from build123d import *

# Parameters (mm, degrees)
SKETCH1_W           = 21.9
SKETCH1_H           = 28.1
BOSS_EXTRUDE1_DEPTH = 1.75
SKETCH2_R           = 1.4
CUT_EXTRUDE1_DEPTH  = 18.89881281
SKETCH3_W           = 5.2
SKETCH3_H           = 5.2
BOSS_EXTRUDE2_DEPTH = 1
SKETCH4_W           = 20.3
SKETCH4_H           = 2.5
BOSS_EXTRUDE3_DEPTH = 2.55
SKETCH5_W           = 0.6
SKETCH5_H           = 0.6
BOSS_EXTRUDE4_DEPTH = 6.1
LPATTERN1_COUNT     = 8
LPATTERN1_PITCH     = 2.54


with BuildPart() as part:
    # Sketch1 → Boss-Extrude1 (new body)
    with BuildSketch(Plane.XY):
        Rectangle(SKETCH1_W, SKETCH1_H)
    extrude(amount=BOSS_EXTRUDE1_DEPTH)

    # Sketch2 → Cut-Extrude1 (cut, through all)
    with BuildSketch(Plane.XY.offset(1.75)):
        with Locations((-9.075, -0.89)):
            Circle(SKETCH2_R)
        with Locations((9.075, -0.89)):
            Circle(SKETCH2_R)
        with Locations((9.075, -12.05)):
            Circle(SKETCH2_R)
        with Locations((-9.075, -12.05)):
            Circle(SKETCH2_R)
    extrude(amount=-CUT_EXTRUDE1_DEPTH, mode=Mode.SUBTRACT)

    # Sketch3 → Boss-Extrude2 (add)
    with BuildSketch(Plane.XY.offset(1.75)):
        with Locations((0, -6.47)):
            Rectangle(SKETCH3_W, SKETCH3_H)
    extrude(amount=BOSS_EXTRUDE2_DEPTH)

    # Sketch4 → Boss-Extrude3 (add)
    with BuildSketch(Plane.XY.offset(1.75)):
        with Locations((0, 12.3)):
            Rectangle(SKETCH4_W, SKETCH4_H)
    extrude(amount=BOSS_EXTRUDE3_DEPTH)

    # Sketch5 → Boss-Extrude4 (add)
    with BuildSketch(Plane.XY.offset(4.3)):
        with Locations((-8.78, 12.3)):
            Rectangle(SKETCH5_W, SKETCH5_H)
    boss_extrude4 = extrude(amount=BOSS_EXTRUDE4_DEPTH)

    # LPattern1: Boss-Extrude4 ×8
    with Locations(*[(i * LPATTERN1_PITCH, 0, 0) for i in range(1, LPATTERN1_COUNT)]):
        add(boss_extrude4)


solid = part.part
Read the model definition and answer for the solid it produces. Units are mm, in the model's axes. A direction names the side the tool comes from. Give positions to 0.01 mm unless a question says otherwise; leave off trailing zeros. Write each loop counter-clockwise with the first axis right and the second up, starting at its lowest first coordinate (ties: lowest second). Pieces come first, ordered by that corner, then holes. Notation, with made-up numbers: (57.25, 3) - (78.25, 3) arc R23 ccw to (78.25, 35) - close; hole circle Ø7 at (9.25, 68.5). An arc over 180 degrees is marked (long way). Use CSV: the item, a comma, the result in double quotes. Start each with the question number.
(1) Find section C-C (z = 8.5). Count the separate pieces of the cut face and the enclosed holes in it, plus the area to 3 significant figures.
(2) Given P1, Ø0.5, axis at y = 12.5, z = 8, coming from the -X side; P2, Ø0.7, axis at y = 12.5, z = 7.5, coming from the +X side; P3, Ø6.5, axis at x = 3.5, y = 3, coming from the +Z side; P4, Ø2.5, axis at x = 9.075, y = -12.05, coming from the -Z side, each flat-ended and moving along its own axis, determine where each tip first touches the part or whether it passes through.
(3) Find section A-A (z = 2.25). Give the vertices of the cut face in (x, y), plus the area to 3 significant figures.
(4) Find section B-B (y = -0.89). Give the vertices of the cut face in (x, z) (3 decimals), plus the area to 3 significant figures.
(5) For faces 4 (the flat face through (0, 13.55, 3)), 5 (the flat face through (2.6, -7, 2)), 6 (the flat face through (0, -9.07, 2)), 7 (the flat face through (0, -3.87, 2)), determine the directions among +Z, -Z, +X, -X, +Y, -Y from which every point of the face is accessible in a straight line to the end or side of a thin tool.
(6) Determine the mould class of faces 1 (the flat face through (0, 0, 1.75)), 2 (the flat face through (0, 14.05, 1)), 3 (the flat face through (0, 12, 4.3)) for opening direction Y: +Y half, -Y half, draft (parallel to the pull), parting line (faces both ways), or undercut.
(7) Consider line 1 along Y through (x, z) = (-1.5, 2); line 2 along Y through (x, z) = (9.5, 1.25); line 3 along Y through (x, z) = (-8.25, 1.5). Determine where each line is inside the solid, lowest interval first.
(8) Find section D-D (z = 0.75). Give the vertices of the cut face in (x, y) (3 decimals), plus the area to 3 significant figures.
Findings below:
1,separate pieces,"8"
1,enclosed holes,"0"
1,area,"2.88 mm2"
2,P1,"x = -9.08"
2,P2,"x = 9.3"
2,P3,"z = 1.75"
2,P4,"through"
3,outline,"(-10.15, 11.05) - (10.15, 11.05) - (10.15, 13.55) - (-10.15, 13.55) - close; (-2.6, -9.07) - (2.6, -9.07) - (2.6, -3.87) - (-2.6, -3.87) - close"
3,area,"77.8 mm2"
4,outline,"(-10.95, 0) - (-10.475, 0) - (-10.475, 1.75) - (-10.95, 1.75) - close; (-7.675, 0) - (7.675, 0) - (7.675, 1.75) - (-7.675, 1.75) - close; (10.475, 0) - (10.95, 0) - (10.95, 1.75) - (10.475, 1.75) - close"
4,area,"28.5 mm2"
5,face 4,"+Z, +X, -X, +Y"
5,face 5,"+Z, +X, -Y"
5,face 6,"+Z, +X, -X, -Y"
5,face 7,"+Z, +X, -X"
6,face 1,"undercut"
6,face 2,"+Y half"
6,face 3,"draft"
7,line 1,"-9.07 to -3.87, 11.05 to 13.55"
7,line 2,"-14.05 to -13.38, -10.72 to -2.22, 0.44 to 14.05"
7,line 3,"-14.05 to -13.18, -10.92 to -2.02, 0.24 to 14.05"
8,outline,"(-10.95, -14.05) - (10.95, -14.05) - (10.95, 14.05) - (-10.95, 14.05) - close; hole circle Ø2.8 at (-9.075, -12.05); hole circle Ø2.8 at (-9.075, -0.89); hole circle Ø2.8 at (9.075, -12.05); hole circle Ø2.8 at (9.075, -0.89)"
8,area,"591 mm2"
